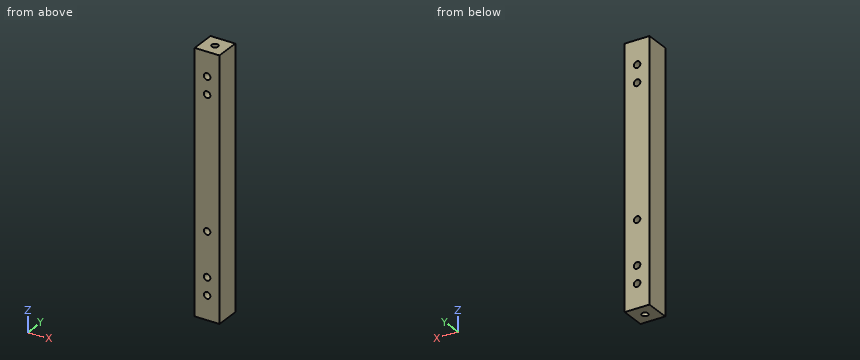
from build123d import *

# Parameters (mm, degrees)
SKETCH_W     = 11.4
SKETCH_H     = 11.4
SKETCH_R     = 1.5
PAD_DEPTH    = 118.85
SKETCH001_R  = 1.5
POCKET_DEPTH = 11.401


with BuildPart() as part:
    # Sketch → Pad (new body)
    with BuildSketch(Plane.XY):
        with Locations((5.7, 5.7)):
            Rectangle(SKETCH_W, SKETCH_H)
        with Locations((5.7, 5.7)):
            Circle(SKETCH_R, mode=Mode.SUBTRACT)
    extrude(amount=PAD_DEPTH)

    # Sketch001 → Pocket (cut, through all)
    with BuildSketch(Plane.XZ):
        with Locations((5.7, 11)):
            Circle(SKETCH001_R)
        with Locations((5.7, 19)):
            Circle(SKETCH001_R)
        with Locations((5.7, 107.85)):
            Circle(SKETCH001_R)
        with Locations((5.7, 99.85)):
            Circle(SKETCH001_R)
        with Locations((5.7, 39.3)):
            Circle(SKETCH001_R)
    extrude(amount=-POCKET_DEPTH, mode=Mode.SUBTRACT)


solid = part.part
The model under review builds one solid part; all positions refer to its coordinate system, in mm. Round coordinates to 2 decimals unless told otherwise and drop trailing zeros. Loops run counter-clockwise (first coordinate to the right, second up) from the corner with the lowest first, then second, coordinate; pieces in that order, holes last. Notation, with made-up numbers: (59, -19) -> (92, -19) arc R7 cw to (92, -9) -> close; hole circle Ø9 at (45, 27.5). An arc over 180 degrees is marked (long way). Return JSON: item names as keys, results as strings.
(1) For pin 1 (2 mm diameter, centred on x = 8, z = 91, fed in from -Y), flat-tipped, find the tip position at first contact; note if it passes through.
Solved:
{"pin 1": "y = 0"}
(2) Add section B-B on z = 92. Write out the cut boundary in (x, y), plus the area to 3 significant figures.
Solved:
{"outline": "(0, 0) -> (11.4, 0) -> (11.4, 11.4) -> (0, 11.4) -> close; hole circle Ø3 at (5.7, 5.7)", "area": "123 mm2"}
(3) For line 1 (Z direction, x = 5.7, y = 10.2); line 2 (X direction, y = 3.95, z = 107.85); line 3 (Z direction, x = 4.5, y = 1), list the stretches that pass through material, from the lowest coordinate up.
Solved:
{"line 1": "0 to 9.5, 12.5 to 17.5, 20.5 to 37.8, 40.8 to 98.35, 101.35 to 106.35, 109.35 to 118.85", "line 2": "0 to 4.2, 7.2 to 11.4", "line 3": "0 to 10.1, 11.9 to 18.1, 19.9 to 38.4, 40.2 to 98.95, 100.75 to 106.95, 108.75 to 118.85"}
(4) Add section C-C on x = 5.7. State how many separate pieces and enclosed holes the cut face has, plus the area to 3 significant figures.
Solved:
{"separate pieces": "12", "enclosed holes": "0", "area": "872 mm2"}
(5) Add section A-A on y = 2.5. Write out the cut boundary in (x, z).
Solved:
{"outline": "(0, 0) -> (11.4, 0) -> (11.4, 118.85) -> (0, 118.85) -> close; hole circle Ø3 at (5.7, 11); hole circle Ø3 at (5.7, 19); hole circle Ø3 at (5.7, 39.3); hole circle Ø3 at (5.7, 99.85); hole circle Ø3 at (5.7, 107.85)"}
